```python
from build123d import *

# Parameters (mm, degrees)
ESBO_O2_R                  = 10.5
ESBO_O2_R_2                = 8.5
CORTE_EXTRUS_O1_DEPTH      = 205.674163986
CORTE_EXTRUS_O1_DEPTH_BACK = 205.674163986
ESBO_O3_R                  = 12.7


with BuildPart() as part:
    # Varredura1: sweep along a path in Esboço1
    with BuildLine(Plane(origin=(0, 0, 0), x_dir=(1, 0, 0), z_dir=(0, 1, 0))) as varredura1_path:
        Line((0, 0), (-122.5, 0))
        Line((-122.5, 0), (-190.5, -47.614112598))
    # Esboço2 → Varredura1 (sweep)
    with BuildSketch(Plane(origin=(0, 0, 0), x_dir=(0, 0, -1), z_dir=(1, 0, 0))):
        Circle(ESBO_O2_R)
        Circle(ESBO_O2_R_2, mode=Mode.SUBTRACT)
    varredura1 = sweep(path=varredura1_path.line, transition=Transition.RIGHT)

    # Espelhar1: Varredura1 across plane
    add(varredura1.mirror(Plane(origin=(0, 0, 0), x_dir=(0, 0, 1), z_dir=(1, 0, 0))))

    # Esboço3 → Corte-extrusão1 (cut, two sides: drawn at the far end of the back side and taken through both)
    with BuildSketch(Plane(origin=(0, 0, 0), x_dir=(1, 0, 0), z_dir=(0, 1, 0)).offset(-CORTE_EXTRUS_O1_DEPTH_BACK)):
        with Locations((196.352209331, -51.711873687)):
            Circle(ESBO_O3_R)
        with Locations((-196.352209331, -51.711873687)):
            Circle(ESBO_O3_R)
    extrude(amount=CORTE_EXTRUS_O1_DEPTH + CORTE_EXTRUS_O1_DEPTH_BACK, mode=Mode.SUBTRACT)


solid = part.part
```
Work out the finished part from the listing and answer in its coordinate system (mm). Round coordinates to 2 decimals unless told otherwise and drop trailing zeros. Write each loop counter-clockwise with the first axis right and the second up, starting at its lowest first coordinate (ties: lowest second). Pieces come first, ordered by that corner, then holes.
1) A cutting plane is placed at C-C on z = 17. Give the number of separate pieces and of enclosed holes in the cut face, and give its area (3 significant figures).
2) Flat-ended cylindrical pins translate along their axes: P1, Ø4, axis at y = -5, z = 35.5, coming from the +X side; P2, Ø6, axis at y = 4, z = 32.5, coming from the +X side; P3, Ø12, axis at y = 3.5, z = 26.5, coming from the -X side. Find the tip coordinate at first contact, or state that the pin passes through.
3) Determine the mould class of faces 1 (the face through (159.6, -2.6, 16.1)), 2 (the face through (161.202, 4.022, 15.259)), 3 (the face through (183.73, 6.18, 50.31)) for opening direction Z: pulls with the +Z half, pulls with the -Z half, needs draft (parallel to the pull), parting line crosses it, or undercut.
4) A cutting plane is placed at B-B on x = 11.5. Determine the outline of the cut face in (y, z), and give its area (3 significant figures).
5) Consider probe 1 along X at (y, z) = (0, 9); probe 2 along X at (y, z) = (0, 29.5); probe 3 along X at (y, z) = (-0.25, 10). Determine where each line is inside the solid, lowest interval first.
6) A cutting plane is placed at A-A on y = 0. Determine the outline of the cut face in (x, z).
Entries:
1. separate pieces: 2
1. enclosed holes: 2
1. area: 416 mm2
2. P1: stops at x = 192.6
2. P2: stops at x = 190.5
2. P3: stops at x = -186.61
3. face 1: undercut
3. face 2: parting line crosses it
3. face 3: undercut
4. outline: circle Ø21 at (0, 0); hole circle Ø17 at (0, 0)
4. area: 119 mm2
5. probe 1: x = -153.66 to -150.17, -120.53 to 120.53, 150.17 to 153.66
5. probe 2: x = -182.94 to -179.45, -149.81 to -146.32, 146.32 to 149.81, 179.45 to 182.94
5. probe 3: x = -155.08 to -151.59, -121.97 to 121.97, 151.59 to 155.08
6. outline: (-196.52, 39.01) - (-125.81, -10.5) - (125.81, -10.5) - (196.52, 39.01) arc R12.7 cw to (193.5, 39.34) - (125.18, -8.5) - (-125.18, -8.5) - (-193.5, 39.34) arc R12.7 cw to start; (-184.48, 56.22) arc R12.7 cw to (-183.75, 53.26) - (-119.82, 8.5) - (119.82, 8.5) - (183.75, 53.26) arc R12.7 cw to (184.48, 56.22) - (119.19, 10.5) - (-119.19, 10.5) - close
